For this review, take the finished solid that the model builds, in its own axes (mm). Give positions to 0.01 mm unless a question says otherwise; leave off trailing zeros. Order: outer loops, then holes, each group sorted by start corner. A loop starts at its lowest first (then second) coordinate and runs counter-clockwise, first axis right, second up.
Item 1: The part is to be moulded in two halves that separate along Y. For faces 1 (the cylindrical face through (-1.526, 1.399, 3.219)), 2 (the flat face through (0, -4.445, 2)), 3 (the flat face through (1, -2, 6.35)), say which applies: released by +Y, released by -Y, zero draft, split by the parting line, or undercut.
Item 2: For probe 1 along Y at (x, z) = (0, 2) (3 decimals); probe 2 along Y at (x, z) = (-0.5, 0.5) (3 decimals); probe 3 along X at (y, z) = (-1.5, 2.25), list the stretches that pass through material, from the lowest coordinate up.
Item 3: For P1, Ø2, axis at x = 3, z = 4.5, coming from the -Y side (3 decimals); P2, Ø3, axis at y = 1.5, z = 5.5, coming from the -X side; P3, Ø1.5, axis at y = -2, z = 5.5, coming from the -X side, all flat-tipped, find the tip position at first contact; note any pin that passes through.
Item 4: Consider section A-A (z = 1). Give the boundary of the cut face in (x, y) (3 decimals), plus the area to 3 significant figures.
Autodesk Inventor part; units mm, degrees
ref_plane "Work Plane1" through (0, 0, 6.35) normal (0, 0, 1) x (1, 0, 0)
ref_plane "YZ Plane" through (0, 0, 0) normal (1, 0, 0) x (0, 1, 0)
ref_plane "XZ Plane" through (0, 0, 0) normal (0, 1, 0) x (-1, 0, 0)
sketch "Sketch1" plane through (0, 0, 0) normal (0, 0, 1) x (1, 0, 0)
  line L0 (2.5663, 4.445) -> (5.1326, 0)
  line L1 (5.1326, 0) -> (2.5663, -4.445)
  line L2 (2.5663, -4.445) -> (-2.5663, -4.445)
  line L3 (-2.5663, -4.445) -> (-5.1326, 0)
  line L4 (-5.1326, 0) -> (-2.5663, 4.445)
  line L5 (-2.5663, 4.445) -> (2.5663, 4.445)
  line L6 (0, 0) -> (0.7817, 0)
  dimension "d0" = 8.89
extrude "Extrusion1" add sketch "Sketch1" along normal blind 3.81
sketch "Sketch2" plane through (0, 0, 3.81) normal (0, 0, 1) x (1, 0, 0)
  line L0 (5.1326, 0) -> (2.5663, 4.445)
  line L1 (2.5663, 4.445) -> (-2.5663, 4.445)
  line L2 (-2.5663, 4.445) -> (-5.1326, 0)
  line L3 (-5.1326, 0) -> (-2.5663, -4.445)
  line L4 (-2.5663, -4.445) -> (2.5663, -4.445)
  line L5 (2.5663, -4.445) -> (5.1326, 0)
  point P0 (0, 0)
ref_plane "Work Plane1" through (0, 0, 6.35) normal (0, 0, 1) x (1, 0, 0)
sketch "Sketch3" plane through (0, 0, 6.35) normal (0, 0, 1) x (1, 0, 0)
  circle A0 centre (0, 0) radius 4.445
  dimension "d4" = 8.89
loft "Loft1" add profiles "Sketch2", "Sketch3"
sketch "Sketch4" plane through (0, 0, 6.35) normal (0, 0, 1) x (1, 0, 0)
  circle A0 centre (0, 0) radius 2.0701
  dimension "d9" = 4.1402
extrude "Extrusion2" cut sketch "Sketch4" against normal blind 25.4
properties part number "RobotArm Nut3"
Resolved:
1. face 1: undercut
1. face 2: released by -Y
1. face 3: zero draft
2. probe 1: y = -4.445 to -2.07, 2.07 to 4.445
2. probe 2: y = -4.445 to -2.009, 2.009 to 4.445
2. probe 3: x = -4.27 to -1.43, 1.43 to 4.27
3. P1: stops at y = -4.445
3. P2: stops at x = -4.8
3. P3: stops at x = -4.32
4. outline: (-5.133, 0) - (-2.566, -4.445) - (2.566, -4.445) - (5.133, 0) - (2.566, 4.445) - (-2.566, 4.445) - close; hole circle Ø4.14 at (0, 0)
4. area: 55.0 mm2
